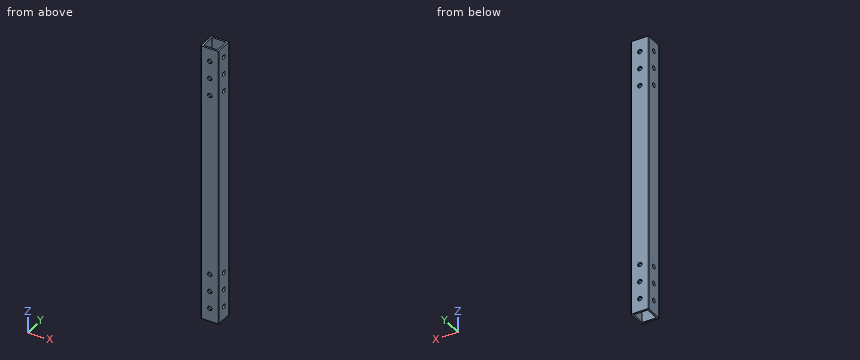
from build123d import *

# Parameters (mm, degrees)
F0_W     = 25.4
F0_H     = 25.4
F0_W_2   = 20.32
F0_H_2   = 20.32
F1_DEPTH = 406.4
F2_R     = 0.762
F5_D     = 6.35
F8_D     = 6.35


with BuildPart() as f1:
    # F0 (on Top) → F1 (new body)
    with BuildSketch(Plane.XY):
        Rectangle(F0_W, F0_H)
        Rectangle(F0_W_2, F0_H_2, mode=Mode.SUBTRACT)
    extrude(amount=F1_DEPTH)

    # F2
    f2_edges = [f1.edges().sort_by_distance(p)[0] for p in [
        (12.7, 12.7, 203.2),
        (-12.7, 12.7, 203.2),
        (-12.7, -12.7, 203.2),
        (12.7, -12.7, 203.2),
    ]]
    fillet(f2_edges, radius=F2_R)

    # F5 (through all)
    with Locations(Plane.YZ.offset(12.7)):
        with Locations((0, 391.16), (0, 365.76), (0, 340.36), (0, 69.85), (0, 44.45), (0, 19.05)):
            Hole(F5_D / 2)

    # F8 (through all)
    with Locations(Plane.XZ.offset(12.7)):
        with Locations((0, 19.05), (0, 44.45), (0, 69.85), (0, 336.55), (0, 361.95), (0, 387.35)):
            Hole(F8_D / 2)


solid = f1.part
Design review of the part built by this model. Coordinates are the model's own, in mm. Round coordinates to 2 decimals unless told otherwise and drop trailing zeros. Write each loop counter-clockwise with the first axis right and the second up, starting at its lowest first coordinate (ties: lowest second). Pieces come first, ordered by that corner, then holes. Notation, with made-up numbers: M 31.25,58 L 89.25,58 A29 cw 89.25,96 Z; hole C 72,76.25 d8. An arc over 180 degrees is marked long. One line per item, written item: value. Start each with the question number.
1. Clearance check with a flat-ended pin moving along its axis: P1, Ø5.5, axis at x = 0, z = 19.05, coming from the -Y side. State where the tip first meets the part, or that it passes through.
2. To check wall thickness, follow probe 1 along X at (y, z) = (-0.25, 318.5); probe 2 along Y at (x, z) = (-10.85, 391.16) (3 decimals). State the ranges of each line that lie inside material, in increasing order. Write a range as from..to.
3. Take a section at A-A on z = 113.5. State the section outline as (x, y) points, then the cut area to 3 significant figures.
Computed:
1. P1: passes through
2. probe 1: x = -12.7..-10.16, 10.16..12.7
2. probe 2: y = -12.7..-3.175, 3.175..12.7
3. outline: M -12.7,-11.94 A0.76 ccw -11.94,-12.7 L 11.94,-12.7 A0.76 ccw 12.7,-11.94 L 12.7,11.94 A0.76 ccw 11.94,12.7 L -11.94,12.7 A0.76 ccw -12.7,11.94 Z; hole M -10.16,-10.16 L 10.16,-10.16 L 10.16,10.16 L -10.16,10.16 Z
3. area: 232 mm²
